The figure shows three views and two pictorial views of one solid part (mm, origin at its lowest corner). Answer the questions. Coordinates: 2 decimals unless noted, no trailing zeros. Order: outer loops, then holes, each group sorted by start corner. A loop starts at its lowest first (then second) coordinate and runs counter-clockwise, first axis right, second up. Notation, with made-up numbers: (-11.5, 20) -> (17.5, 20) arc R9 cw to (17.5, 35) -> close; hole circle Ø3 at (27, 8.25). An arc over 180 degrees is marked (long way). Use one line per item in the form item = value.
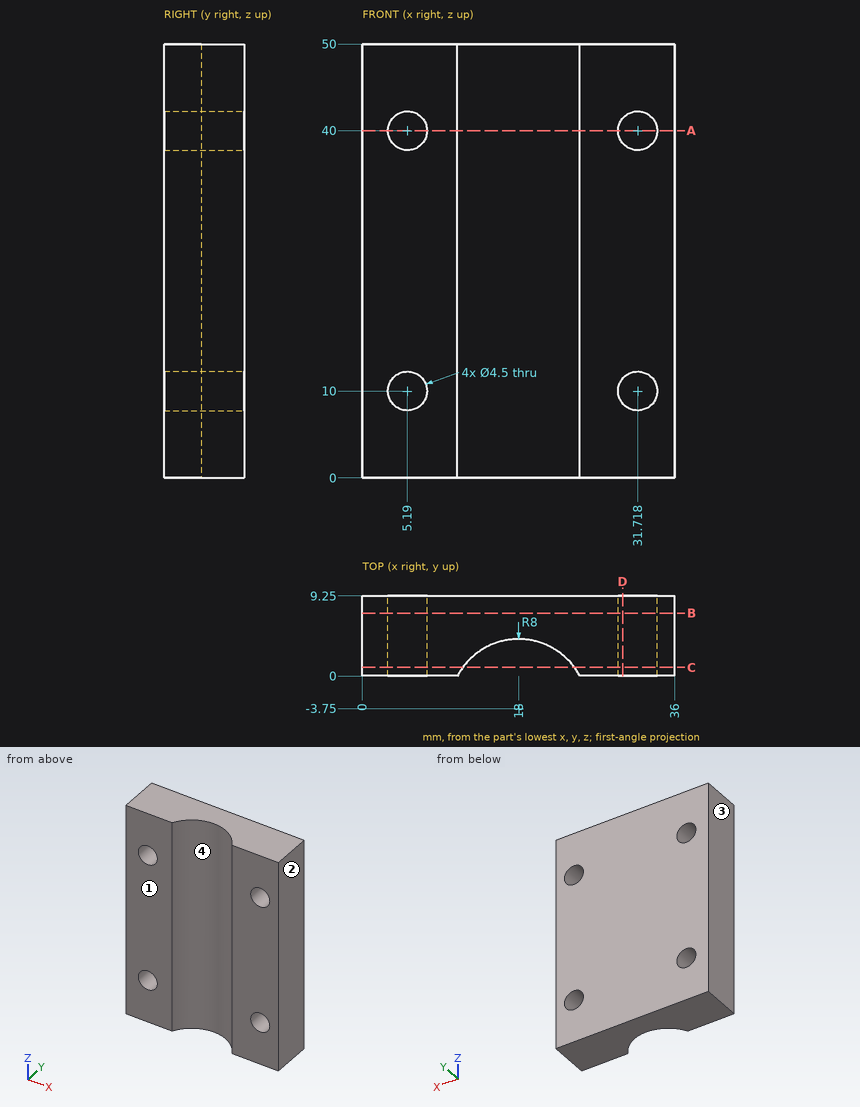
(1) Section D-D on x = 30 is taken. Write down the section's boundary in (y, z).
Data:
outline = (0, 0) -> (9.25, 0) -> (9.25, 8.55) -> (0, 8.55) -> close; (0, 11.45) -> (9.25, 11.45) -> (9.25, 38.55) -> (0, 38.55) -> close; (0, 41.45) -> (9.25, 41.45) -> (9.25, 50) -> (0, 50) -> close
(2) Section A-A on z = 40 is taken. Write down the section's boundary in (x, y).
Data:
outline = (0, 0) -> (2.94, 0) -> (2.94, 9.25) -> (0, 9.25) -> close; (7.44, 0) -> (10.93, 0) arc R8 cw to (25.07, 0) -> (29.47, 0) -> (29.47, 9.25) -> (7.44, 9.25) -> close; (33.97, 0) -> (36, 0) -> (36, 9.25) -> (33.97, 9.25) -> close
(3) Section B-B on y = 7.25 is taken. Write down the section's boundary in (x, z), plus the area to 3 significant figures.
Data:
outline = (0, 0) -> (36, 0) -> (36, 50) -> (0, 50) -> close; hole circle Ø4.5 at (5.19, 10); hole circle Ø4.5 at (5.19, 40); hole circle Ø4.5 at (31.72, 10); hole circle Ø4.5 at (31.72, 40)
area = 1,740 mm²
(4) Section C-C on y = 1 is taken. Write down the section's boundary in (x, z), plus the area to 3 significant figures.
Data:
outline = (0, 0) -> (11.56, 0) -> (11.56, 50) -> (0, 50) -> close; (24.44, 0) -> (36, 0) -> (36, 50) -> (24.44, 50) -> close; hole circle Ø4.5 at (5.19, 10); hole circle Ø4.5 at (5.19, 40); hole circle Ø4.5 at (31.72, 10); hole circle Ø4.5 at (31.72, 40)
area = 1,090 mm²
(5) The mould has two halves that part along X. Classify the marked faces 1, 2, 3 and 4: released by +X, released by -X, zero draft, split by the parting line, or undercut.
Data:
face_1 = zero draft
face_2 = released by +X
face_3 = released by -X
face_4 = undercut
(6) Straight lines are drawn through the part: line 1 along X through (y, z) = (6.5, 10); line 2 along X through (y, z) = (3.25, 10) (1 decimal); line 3 along Z through (x, y) = (7, 6) (1 decimal). For each, find the intervals that lie inside material, in ascending order.
Data:
line_1 = 0 to 2.94, 7.44 to 29.47, 33.97 to 36
line_2 = 0 to 2.9, 7.4 to 14.1, 21.9 to 29.5, 34 to 36
line_3 = 0 to 8.7, 11.3 to 38.7, 41.3 to 50
